Verification items for the finished model (mm, model axes). A direction names the side the tool comes from. Round coordinates to 2 decimals unless told otherwise and drop trailing zeros. Order: outer loops, then holes, each group sorted by start corner. A loop starts at its lowest first (then second) coordinate and runs counter-clockwise, first axis right, second up. Notation, with made-up numbers: (-5, 53.25) -> (20, 53.25) arc R22 cw to (20, 88.25) -> close; hole circle Ø11 at (81, 12.5). An arc over 180 degrees is marked (long way). Write item = value, one per line. Start each with the question number.
from build123d import *

# Parameters (mm, degrees)
F1_DEPTH = 56
F2_R     = 0.99999


# Not quite as in the source:
# - a fillet or chamfer is up to 0.001 mm smaller than in the source, because OpenCascade refuses the exact size


with BuildPart() as f1:
    # F0 (on Right) → F1 (new body)
    with BuildSketch(Plane.YZ):
        Polygon((0, 0), (14.5, 0), (14.5, 1), (13.5, 1), (13.5, 2), (0, 2), (-6.25, 2), (-13.5, 2), (-13.5, 1), (-14.5, 1), (-14.5, 0), (-7.25, 0), align=None)
    extrude(amount=F1_DEPTH)

    # F2 (radius 1 in the source; OpenCascade refuses exactly that, so slightly less here)
    f2_edges = [f1.edges().sort_by_distance(p)[0] for p in [
        (28, 13.5, 2),
        (28, -13.5, 2),
        (28, 14.5, 0),
        (28, -14.5, 0),
        (0, 0, 2),
        (0, 0, 0),
    ]]
    fillet(f2_edges, radius=F2_R)


solid = f1.part
(1) Cross-section at B-B (z = 1.4). Enter the section's corners in (x, y).
(2) Scan lines: line 1 along X through (y, z) = (9.75, 1.1); line 2 along Y through (x, z) = (50, 1.05); line 3 along Y through (x, z) = (51, 0.75). Record each from-to range of solid material in increasing order. Write a range as from..to.
(3) Set-up check for faces 1 (the flat face through (28, -14, 1)), 2 (the flat face through (28, 14, 1)), 3 (the cylindrical face through (28.392, -14.215, 0.301)): record each of +Z, -Z, +X, -X, +Y, -Y from which the full face is reachable in a straight line by a thin tool's end or side.
Outcome:
q1.outline = (0.08, -13.42) -> (56, -13.42) -> (56, 13.42) -> (0.08, 13.42) -> close
q2.line_1 = 0.01..56
q2.line_2 = -13.5..13.5
q2.line_3 = -14.47..14.47
q3.face_1 = +Z, +X, -X, -Y
q3.face_2 = +Z, +X, -X, +Y
q3.face_3 = -Z, +X, -X, -Y
